The listing builds one solid part. Answer for the finished solid, in the listing's coordinates (mm). A direction names the side the tool comes from. Coordinates: 2 decimals unless noted, no trailing zeros. Order: outer loops, then holes, each group sorted by start corner. A loop starts at its lowest first (then second) coordinate and runs counter-clockwise, first axis right, second up.
from build123d import *

# Parameters (mm, degrees)
F6_W      = 114
F6_H      = 132.5
F7_DEPTH  = 0.6
F5_W      = 152.5
F5_H      = 114
F9_DEPTH  = 0.6
F1_W      = 152.5
F1_H      = 132.5
F10_DEPTH = 0.6
F3_W      = 152.5
F3_H      = 132.5
F11_DEPTH = 0.6
F0_W      = 152.5
F0_H      = 114
F12_DEPTH = 0.6
F13_W     = 152.5
F13_H     = 132.5
F14_DEPTH = 25
F16_DEPTH = 7
F18_DEPTH = 7.6


with BuildPart() as f7:
    # F6 (on Right) → F7 (new body)
    with BuildSketch(Plane.YZ):
        with Locations((57, 66.25)):
            Rectangle(F6_W, F6_H)
    extrude(amount=F7_DEPTH)

    # F5 (on line) → F9 (join)
    with BuildSketch(Plane.XY.offset(132.5)):
        with Locations((76.25, 57)):
            Rectangle(F5_W, F5_H)
    extrude(amount=-F9_DEPTH)

    # F1 (on Front) → F10 (join)
    with BuildSketch(Plane.XZ):
        with Locations((76.25, 66.25)):
            Rectangle(F1_W, F1_H)
    extrude(amount=-F10_DEPTH)

    # F3 (on line) → F11 (join)
    with BuildSketch(Plane(origin=(0, 114, 0), x_dir=(-1, 0, 0), z_dir=(0, 1, 0))):
        with Locations((-76.25, 66.25)):
            Rectangle(F3_W, F3_H)
    extrude(amount=-F11_DEPTH)

    # F0 (on Top) → F12 (join)
    with BuildSketch(Plane.XY):
        with Locations((76.25, 57)):
            Rectangle(F0_W, F0_H)
    extrude(amount=F12_DEPTH)

    # F13 (on face) → F14 (join)
    with BuildSketch(Plane(origin=(0, 114, 0), x_dir=(-1, 0, 0), z_dir=(0, 1, 0))):
        with Locations((-76.25, 66.25)):
            Rectangle(F13_W, F13_H)
    extrude(amount=F14_DEPTH)

    # F15 (on face) → F16 (join)
    with BuildSketch(Plane.XY.offset(132.5)):
        Polygon((0, 94.5), (0, 20), (152.5, 20), (152.5, 42.25), (10.7762217522, 42.25), (10.7762217522, 72.25), (152.5, 72.25), (152.5, 94.5), align=None)
    extrude(amount=F16_DEPTH)

    # F17 (on face) → F18 (join)
    with BuildSketch(Plane(origin=(0, 0, 0), x_dir=(1, 0, 0), z_dir=(0, 0, -1))):
        Polygon((152.5, -25.5), (152.5, 0), (0, 0), (-21, 0), (-21, -12.25), (0, -19.2), (0, -25.5), align=None)
        Polygon((0, -114), (152.5, -114), (152.5, -88.5), (0, -88.5), (0, -94.8), (-21, -101.75), (-21, -114), align=None)
    extrude(amount=F18_DEPTH)


solid = f7.part
(1) Find section C-C on z = 75. Determine the outline of the cut face in (x, y).
(2) Given pin 1 Ø8 at (y, z) = (15.5, 26.5) entering from -X; pin 2 Ø9 at (x, y) = (52, 50.5) entering from +Z; pin 3 Ø8 at (y, z) = (23, 51.5) entering from +X, each flat-ended and moving along its own axis, determine where each tip first touches the part or whether it passes through.
(3) A tool of negligible diameter and unlimited length cuts with its end or side. For faces 1 (the flat face through (75, 20, 136)), 2 (the flat face through (77, 88.5, -4)), 3 (the flat face through (-11, 106, 0)), 4 (the flat face through (75, 58, 0.6)), from which of +Z, -Z, +X, -X, +Y, -Y can it reach the whole face along a straight path? Write none if from no direction.
(4) Find section D-D on y = 58.5. Determine the outline of the cut face in (x, z), then the cut area to 3 significant figures.
(5) Find the intervals of material crossed by probe 1 along Y at (x, z) = (16, 40); probe 2 along Z at (x, y) = (31, 93); probe 3 along Z at (x, y) = (62, 74), in increasing order.
(6) Find section B-B on y = 28.5. Determine the outline of the cut face in (x, z), then the cut area to 3 significant figures.
(7) The mould has two halves that part along Y. Classify faces 5 (the flat face through (65, 13, -7.6)), 6 (the flat face through (77, 94.5, 136)), 7 (the flat face through (83, 57, 132.5)): pulls with the +Y half, pulls with the -Y half, needs draft (parallel to the pull), parting line crosses it, or undercut.
(8) Find section A-A on x = 13. Determine the outline of the cut face in (y, z), then the cut area to 3 significant figures.
Resolved:
1. outline: (0, 0) - (152.5, 0) - (152.5, 0.6) - (0.6, 0.6) - (0.6, 113.4) - (152.5, 113.4) - (152.5, 139) - (0, 139) - close
2. pin 1: stops at x = 0
2. pin 2: stops at z = 132.5
2. pin 3: stops at x = 0.6
3. face 1: +Z, +X, -X, -Y
3. face 2: -Z, +X, -X
3. face 3: +Z, -X, +Y, -Y
3. face 4: +X
4. outline: (0, 0) - (152.5, 0) - (152.5, 0.6) - (0.6, 0.6) - (0.6, 131.9) - (152.5, 131.9) - (152.5, 132.5) - (10.78, 132.5) - (10.78, 139.5) - (0, 139.5) - close
4. area: 337 mm2
5. probe 1: y = 0 to 0.6, 113.4 to 139
5. probe 2: z = -7.6 to 0.6, 131.9 to 139.5
5. probe 3: z = 0 to 0.6, 131.9 to 139.5
6. outline: (0, 0) - (152.5, 0) - (152.5, 0.6) - (0.6, 0.6) - (0.6, 131.9) - (152.5, 131.9) - (152.5, 139.5) - (0, 139.5) - close
6. area: 1,330 mm2
7. face 5: needs draft
7. face 6: pulls with the +Y half
7. face 7: undercut
8. outline: (0, -7.6) - (25.5, -7.6) - (25.5, 0) - (88.5, 0) - (88.5, -7.6) - (114, -7.6) - (114, 0) - (139, 0) - (139, 132.5) - (94.5, 132.5) - (94.5, 139.5) - (72.25, 139.5) - (72.25, 132.5) - (42.25, 132.5) - (42.25, 139.5) - (20, 139.5) - (20, 132.5) - (0, 132.5) - close; hole (0.6, 0.6) - (113.4, 0.6) - (113.4, 131.9) - (0.6, 131.9) - close
8. area: 4,310 mm2
